Check sheet for the drawn part. Datum: minimum x, y, z corner. Units: mm. A direction names the side the tool comes from. Give positions to 0.01 mm unless a question says otherwise; leave off trailing zeros. Loops run counter-clockwise (first coordinate to the right, second up) from the corner with the lowest first, then second, coordinate; pieces in that order, holes last. Notation, with made-up numbers: M -11.5,-6.75 L 39.5,-6.75 A20 ccw 39.5,24.25 Z; hole C 6,-0.5 d4. An arc over 180 degrees is marked long. Write each question's results on one line, items separated by ' | '. Start each with the question number.
1. Sectioned sample at B-B on x = 5. Record the cut outline in (y, z).
2. Draft check along X on the marked faces 1, 2 and 3. Enter one of: pulls with the +X half, pulls with the -X half, needs draft (parallel to the pull), parting line crosses it, or undercut.
3. Material ranges on line 1 along X through (y, z) = (5, 42); line 2 along Z through (x, y) = (59.5, 39.5), recorded low to high.
4. Sectioned sample at A-A on z = 35. Record the cut outline in (x, y), and give its area (3 significant figures).
5. Sectioned sample at C-C on y = 71.5. Record the cut outline in (x, z), and give its area (3 significant figures).
6. Sectioned sample at D-D on z = 7. Record the cut outline in (x, y), and give its area (3 significant figures).
7. Tool access check on the marked faces 4, 5 and 6. Record the directions out of +Z, -Z, +X, -X, +Y, -Y that give a thin tool (end or side, any length) a straight path to the whole face; none if there is none.
8. Go/stop test with flat-tipped pins: pin 1 (23 mm diameter, centred on x = 41, y = 37, fed in from -Z); pin 2 (20.5 mm diameter, centred on x = 70, y = 65, fed in from -Z); pin 3 (12.5 mm diameter, centred on x = 14.5, y = 64.5, fed in from -Z). Record where each tip stops, or that it passes through.
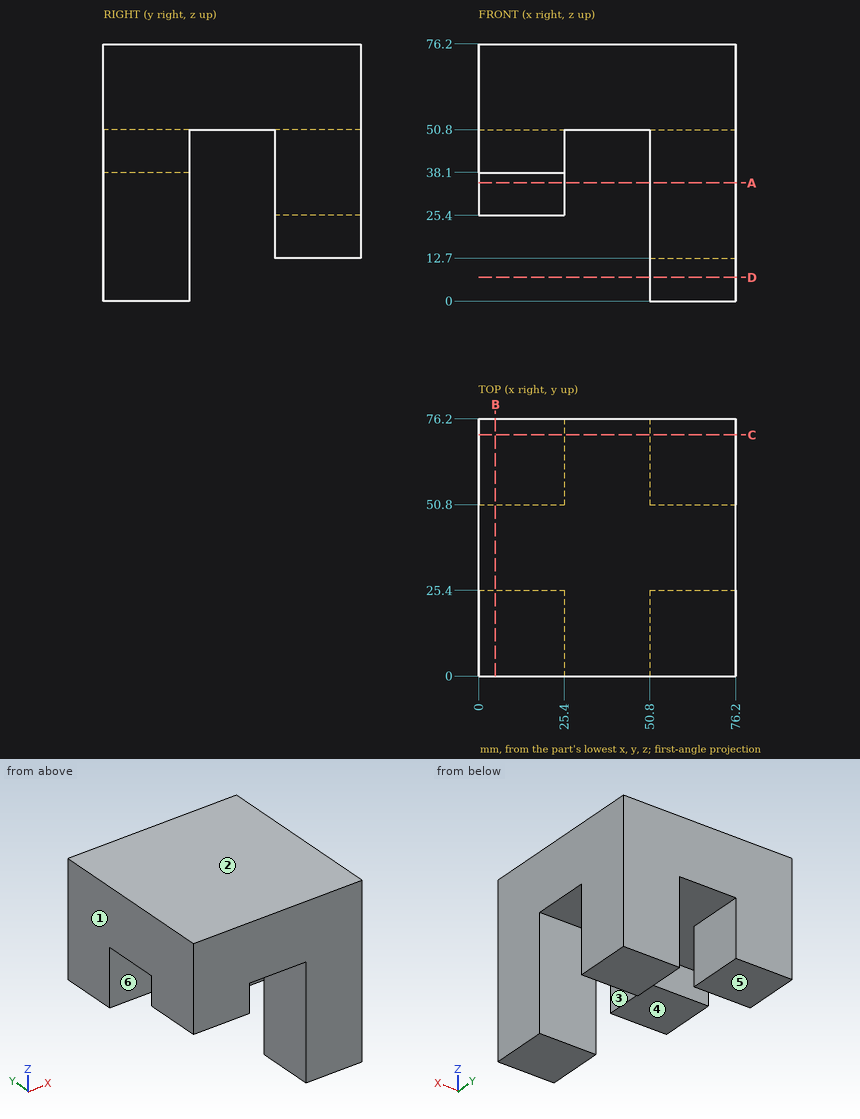
Output values:
1) outline: M 0,38.1 L 25.4,38.1 L 25.4,50.8 L 50.8,50.8 L 50.8,25.4 L 76.2,25.4 L 76.2,76.2 L 0,76.2 Z
2) face 1: pulls with the -X half | face 2: needs draft | face 3: undercut
3) line 1: 0 to 25.4, 50.8 to 76.2 | line 2: 50.8 to 76.2
4) outline: M 0,50.8 L 25.4,50.8 L 25.4,76.2 L 0,76.2 Z; M 50.8,0 L 76.2,0 L 76.2,25.4 L 50.8,25.4 Z; M 50.8,50.8 L 76.2,50.8 L 76.2,76.2 L 50.8,76.2 Z | area: 1,940 mm2
5) outline: M 0,25.4 L 25.4,25.4 L 25.4,50.8 L 50.8,50.8 L 50.8,12.7 L 76.2,12.7 L 76.2,76.2 L 0,76.2 Z | area: 3,550 mm2
6) outline: M 50.8,0 L 76.2,0 L 76.2,25.4 L 50.8,25.4 Z | area: 645 mm2
7) face 4: -Z, -X, -Y | face 5: -Z, -X, +Y, -Y | face 6: -Z, +X, -X
8) pin 1: z = 50.8 | pin 2: z = 12.7 | pin 3: z = 25.4
